Check sheet for the modelled part. Datum: model origin and axes. Units: mm. A direction names the side the tool comes from. Coordinates: 2 decimals unless noted, no trailing zeros. Order: outer loops, then holes, each group sorted by start corner. A loop starts at its lowest first (then second) coordinate and runs counter-clockwise, first axis right, second up. Notation, with made-up numbers: M -23,-29.75 L 33,-29.75 A18 ccw 33,-1.75 Z; hole C 72,-29.75 d4. An arc over 180 degrees is marked long. Answer in a Markdown table with one row per item. Add a question column.
from build123d import *

# Parameters (mm, degrees)
SKETCH1_W               = 36
SKETCH1_H               = 40
SKETCH1_R               = 2
SKETCH1_R_2             = 7.05
BOSS_EXTRUDE1_DEPTH     = 10
BOSS_EXTRUDE2_DEPTH     = 10
FILLET1_R               = 5
CUT_EXTRUDE1_DEPTH      = 36.832945734
CUT_EXTRUDE1_DEPTH_BACK = 36.832945734
SKETCH4_W               = 1
SKETCH4_H               = 8
CUT_EXTRUDE2_REACH      = 53.147
SKETCH5_R               = 1.6


with BuildPart() as part:
    # Sketch1 → Boss-Extrude1 (new body)
    with BuildSketch(Plane(origin=(0, 0, 0), x_dir=(1, 0, 0), z_dir=(0, 1, 0))):
        Rectangle(SKETCH1_W, SKETCH1_H)
        with Locations(Location((-13, 13, 0), (0, 0, 270))):
            Circle(SKETCH1_R, mode=Mode.SUBTRACT)
        with Locations(Location((13, 13, 0), (0, 0, 90))):
            Circle(SKETCH1_R, mode=Mode.SUBTRACT)
        with Locations(Location((-13, -13, 0), (0, 0, 90))):
            Circle(SKETCH1_R, mode=Mode.SUBTRACT)
        with Locations(Location((13, -13, 0), (0, 0, 270))):
            Circle(SKETCH1_R, mode=Mode.SUBTRACT)
        with Locations(Location((0, 0, 0), (0, 0, 270))):
            Circle(SKETCH1_R_2, mode=Mode.SUBTRACT)
    extrude(amount=BOSS_EXTRUDE1_DEPTH)

    # Sketch3 → Boss-Extrude2 (add)
    with BuildSketch(Plane(origin=(0, 0, 0), x_dir=(1, 0, 0), z_dir=(0, 1, 0))):
        Polygon((18, 20), (18, -20), (28, -10), (28, 10), align=None)
    extrude(amount=BOSS_EXTRUDE2_DEPTH)

    # Fillet1
    fillet1_edges = [part.edges().sort_by_distance(p)[0] for p in [
        (28, 5, 10),
        (28, 5, -10),
        (18, 5, 20),
        (-18, 5, 20),
        (-18, 5, -20),
        (18, 5, -20),
    ]]
    fillet(fillet1_edges, radius=FILLET1_R)

    # Sketch4 → Cut-Extrude1 (cut, two sides: drawn at the far end of the back side and taken through both)
    with BuildSketch(Plane.XY.offset(-CUT_EXTRUDE1_DEPTH_BACK)):
        with Locations((22.95, 4)):
            Rectangle(SKETCH4_W, SKETCH4_H)
    extrude(amount=CUT_EXTRUDE1_DEPTH + CUT_EXTRUDE1_DEPTH_BACK, mode=Mode.SUBTRACT)

    # Sketch5 → Cut-Extrude2 (cut, up to next)
    with BuildSketch(Plane(origin=(28, 0, 0), x_dir=(0, 0, -1), z_dir=(1, 0, 0)), mode=Mode.PRIVATE) as cut_extrude2_sk1:
        with Locations((-3.5, 5)):
            Circle(SKETCH5_R)
    cut_extrude2_tool1 = extrude(cut_extrude2_sk1.sketch, amount=-CUT_EXTRUDE2_REACH, mode=Mode.PRIVATE) & part.part
    # Sketch5 → Cut-Extrude2 (cut, up to next)
    with BuildSketch(Plane(origin=(28, 0, 0), x_dir=(0, 0, -1), z_dir=(1, 0, 0)), mode=Mode.PRIVATE) as cut_extrude2_sk2:
        with Locations((3.5, 5)):
            Circle(SKETCH5_R)
    cut_extrude2_tool2 = extrude(cut_extrude2_sk2.sketch, amount=-CUT_EXTRUDE2_REACH, mode=Mode.PRIVATE) & part.part
    add(cut_extrude2_tool1.solids().sort_by_distance((28, 5, 3.5))[0], mode=Mode.SUBTRACT)
    add(cut_extrude2_tool2.solids().sort_by_distance((28, 5, -3.5))[0], mode=Mode.SUBTRACT)


solid = part.part
1. Section check B-B on z = 0. Enter the section's corners in (x, y).
2. Set-up check for faces 4 (the cylindrical face through (25.76, 3.44, -3.15)), 5 (the flat face through (23, 8, 0)), 6 (the cylindrical face through (17.87, 5.07, 19.61)): record each of +Z, -Z, +X, -X, +Y, -Y from which the full face is reachable in a straight line by a thin tool's end or side.
3. Section check D-D on x = 0. Enter the section's corners in (y, z).
4. Scan lines: line 1 (X direction, y = 5, z = 13); line 2 (X direction, y = 3.5, z = 2); line 3 (X direction, y = 2.25, z = 8). Record each from-to range of solid material in increasing order.
5. Section check A-A on x = 13. Enter the section's corners in (y, z).
6. Release check for a two-part mould opening along X. For faces 1 (the flat face through (6, 0, 4)), 2 (the cylindrical face through (-17, 5, -18)), 3 (the cylindrical face through (14.352, 4.93, 11.526)) record: released by +X, released by -X, zero draft, split by the parting line, or undercut.
7. Go/stop test with flat-tipped pins: pin 1 Ø1 at (y, z) = (8.5, -13) entering from +X; pin 2 Ø1.9 at (y, z) = (5, -3.5) entering from +X. Record where each tip stops, or that it passes through.
8. Section check C-C on y = 8.5. Enter the section's corners in (x, z).
Result sheet:
| question | item | result |
|---|---|---|
| 1 | outline | M -18,0 L -7.05,0 L -7.05,10 L -18,10 Z; M 7.05,0 L 22.45,0 L 22.45,8 L 23.45,8 L 23.45,0 L 28,0 L 28,10 L 7.05,10 Z |
| 2 | face 4 | +X |
| 2 | face 5 | +Z, -Z, -Y |
| 2 | face 6 | +Z, +X, +Y, -Y |
| 3 | outline | M 0,-20 L 10,-20 L 10,-7.05 L 0,-7.05 Z; M 0,7.05 L 10,7.05 L 10,20 L 0,20 Z |
| 4 | line 1 | -18 to -15, -11 to 11, 15 to 22.45, 23.45 to 25 |
| 4 | line 2 | -18 to -6.76, 6.76 to 22.45, 23.45 to 28 |
| 4 | line 3 | -18 to 22.45, 23.45 to 28 |
| 5 | outline | M 0,-20 L 10,-20 L 10,-15 L 0,-15 Z; M 0,-11 L 10,-11 L 10,11 L 0,11 Z; M 0,15 L 10,15 L 10,20 L 0,20 Z |
| 6 | face 1 | zero draft |
| 6 | face 2 | released by -X |
| 6 | face 3 | undercut |
| 7 | pin 1 | x = 25.5 |
| 7 | pin 2 | x = 22.45 |
| 8 | outline | M -18,-15 A5 ccw -13,-20 L 15.93,-20 A5 ccw 19.46,-18.54 L 26.54,-11.46 A5 ccw 28,-7.93 L 28,7.93 A5 ccw 26.54,11.46 L 19.46,18.54 A5 ccw 15.93,20 L -13,20 A5 ccw -18,15 Z; hole C -13,-13 d4; hole C -13,13 d4; hole C 0,0 d14.1; hole C 13,-13 d4; hole C 13,13 d4 |
